Answer from the drawing. Dimensions are ordinates in mm from the lowest x, y and z of the part. A direction names the side the tool comes from. Coordinates: 2 decimals unless noted, no trailing zeros. Order: outer loops, then holes, each group sorted by start corner. A loop starts at its lowest first (then second) coordinate and runs counter-clockwise, first axis right, second up. Notation, with made-up numbers: (33, 43.5) -> (86, 43.5) arc R36 ccw to (86, 81.5) -> close; hole circle Ø3 at (-20, -20.5). An arc over 180 degrees is marked (long way). Answer in a Markdown table with one row per item.
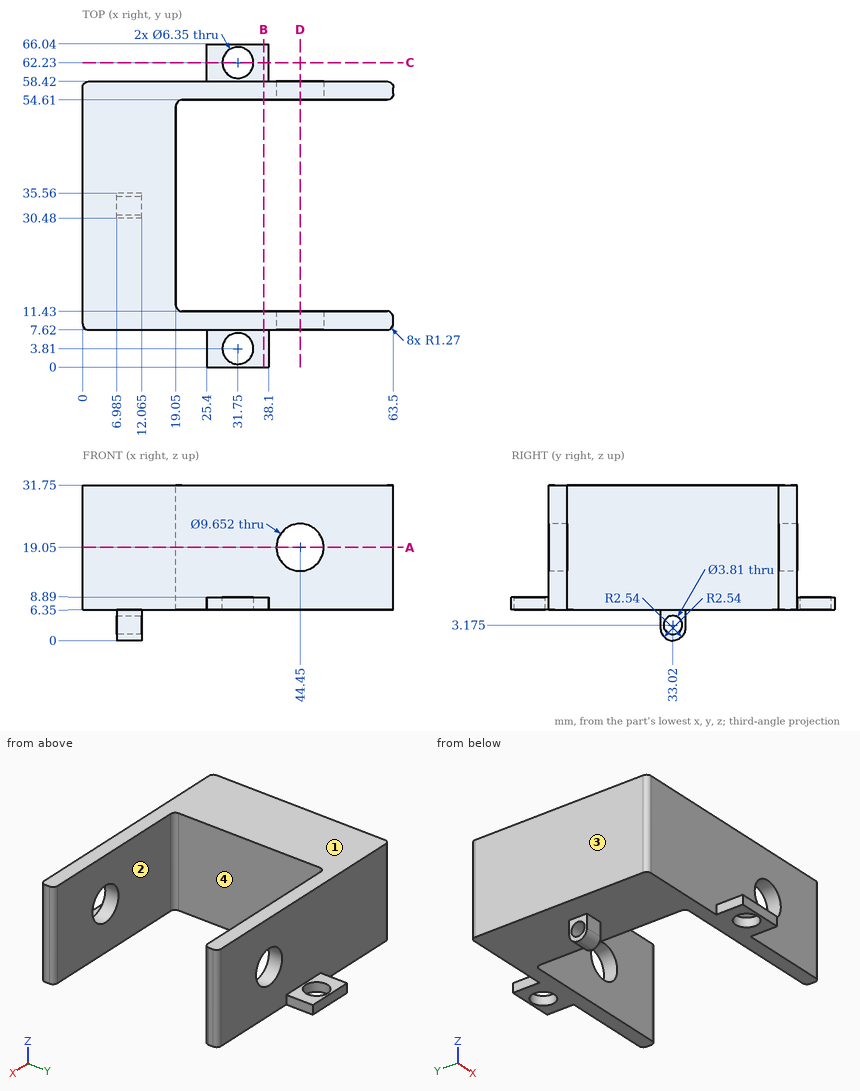
(1) A cutting plane is placed at C-C, the plane y = 62.23. Determine the outline of the cut face in (x, z) (3 decimals).
Check values:
| item | result |
|---|---|
| outline | (25.4, 6.35) -> (28.575, 6.35) -> (28.575, 8.89) -> (25.4, 8.89) -> close; (34.925, 6.35) -> (38.1, 6.35) -> (38.1, 8.89) -> (34.925, 8.89) -> close |
(2) A cutting plane is placed at A-A, the plane z = 19.05. Determine the outline of the cut face in (x, y), then the cut area to 3 significant figures.
Check values:
| item | result |
|---|---|
| outline | (0, 8.89) arc R1.27 ccw to (1.27, 7.62) -> (39.62, 7.62) -> (39.62, 11.43) -> (20.32, 11.43) arc R1.27 cw to (19.05, 12.7) -> (19.05, 53.34) arc R1.27 cw to (20.32, 54.61) -> (39.62, 54.61) -> (39.62, 58.42) -> (1.27, 58.42) arc R1.27 ccw to (0, 57.15) -> close; (49.28, 7.62) -> (62.23, 7.62) arc R1.27 ccw to (63.5, 8.89) -> (63.5, 10.16) arc R1.27 ccw to (62.23, 11.43) -> (49.28, 11.43) -> close; (49.28, 54.61) -> (62.23, 54.61) arc R1.27 ccw to (63.5, 55.88) -> (63.5, 57.15) arc R1.27 ccw to (62.23, 58.42) -> (49.28, 58.42) -> close |
| area | 1,230 mm² |
(3) Which of the six approach directions +Z, -Z, +X, -X, +Y, -Y give full straight-line access (tool end or side, diameter ignored) to the marked faces 3 and 4?
Check values:
| item | result |
|---|---|
| face 3 | +Z, -Z, -X, +Y, -Y |
| face 4 | +Z, -Z, +X |
(4) Find the intervals of material crossed by line 1 along Y through (x, z) = (49, 29); line 2 along Y through (x, z) = (31.5, 7.5) (3 decimals); line 3 along Z through (x, y) = (8, 33), in increasing order. Write a range as from..to.
Check values:
| item | result |
|---|---|
| line 1 | 7.62..11.43, 54.61..58.42 |
| line 2 | 0..0.645, 6.975..11.43, 54.61..59.065, 65.395..66.04 |
| line 3 | 0..1.27, 5.08..31.75 |
(5) Flat-ended cylindrical pins translate along their axes: pin 1 (1.9 mm diameter, centred on x = 10.5, z = 5, fed in from +Y); pin 2 (1 mm diameter, centred on x = 16.5, y = 23.5, fed in from -Z); pin 3 (1.1 mm diameter, centred on x = 10, z = 4.5, fed in from -Y). Find the tip coordinate at first contact, or state that the pin passes through.
Check values:
| item | result |
|---|---|
| pin 1 | y = 35.56 |
| pin 2 | z = 6.35 |
| pin 3 | y = 30.48 |
(6) A cutting plane is placed at D-D, the plane x = 44.45. Determine the outline of the cut face in (y, z).
Check values:
| item | result |
|---|---|
| outline | (7.62, 6.35) -> (11.43, 6.35) -> (11.43, 14.22) -> (7.62, 14.22) -> close; (7.62, 23.88) -> (11.43, 23.88) -> (11.43, 31.75) -> (7.62, 31.75) -> close; (54.61, 6.35) -> (58.42, 6.35) -> (58.42, 14.22) -> (54.61, 14.22) -> close; (54.61, 23.88) -> (58.42, 23.88) -> (58.42, 31.75) -> (54.61, 31.75) -> close |
(7) For a pull along Y with two mould halves and no side action, classify the marked faces 1 and 2 as released by +Y, released by -Y, zero draft, split by the parting line, or undercut.
Check values:
| item | result |
|---|---|
| face 1 | zero draft |
| face 2 | undercut |
(8) A cutting plane is placed at B-B, the plane x = 37. Determine the outline of the cut face in (y, z).
Check values:
| item | result |
|---|---|
| outline | (0, 6.35) -> (11.43, 6.35) -> (11.43, 31.75) -> (7.62, 31.75) -> (7.62, 8.89) -> (0, 8.89) -> close; (54.61, 6.35) -> (66.04, 6.35) -> (66.04, 8.89) -> (58.42, 8.89) -> (58.42, 31.75) -> (54.61, 31.75) -> close |
